Geometry: final body of the model. Coordinates: model frame, mm. A direction names the side the tool comes from. Coordinates: 2 decimals unless noted, no trailing zeros. Loops run counter-clockwise (first coordinate to the right, second up) from the corner with the lowest first, then second, coordinate; pieces in that order, holes last. Notation, with made-up numbers: (35, 47) -> (78, 47) arc R12 ccw to (78, 62) -> close; hole circle Ø2 at (25.5, 1.5). An arc over 180 degrees is marked (long way). One line per item, written item: value. Start each with the question number.
from build123d import *

# Parameters (mm, degrees)
F0_R     = 67.691
F1_DEPTH = 98.298
F2_R     = 76.523192
F3_DEPTH = 228.6


with BuildPart() as f1:
    # F0 (on Top) → F1 (new body)
    with BuildSketch(Plane.XY):
        Polygon((20.642572, -144.15397), (135.162286, -54.199993), (114.519714, 89.953977), (-20.642572, 144.15397), (-135.162286, 54.199993), (-114.519714, -89.953977), align=None)
        Circle(F0_R, mode=Mode.SUBTRACT)
    extrude(amount=F1_DEPTH)

    # F2 (on Top) → F3 (join)
    with BuildSketch(Plane.XY):
        with BuildLine():
            ThreePointArc((246.963915, -59.370235), (252.234845, -29.892856), (254, 0))
            ThreePointArc((254, 0), (251.607755, 34.778404), (244.476083, 68.901703))
            ThreePointArc((244.476083, 68.901703), (227.114105, 77.709336), (235.441325, 95.306781))
            ThreePointArc((235.441325, 95.306781), (203.739291, 151.678282), (158.82823, 198.216027))
            ThreePointArc((158.82823, 198.216027), (139.581788, 195.285642), (136.12364, 214.444293))
            ThreePointArc((136.12364, 214.444293), (77.552803, 241.870963), (13.953987, 253.616416))
            ThreePointArc((13.953987, 253.616416), (0, 240.040742), (-13.953987, 253.616416))
            ThreePointArc((-13.953987, 253.616416), (-86.873116, 238.681926), (-152.332115, 203.250896))
            ThreePointArc((-152.332115, 203.250896), (-150.086276, 199.168943), (-149.308795, 194.575289))
            ThreePointArc((-149.308795, 194.575289), (-158.313913, 181.524718), (-173.710864, 185.311996))
            ThreePointArc((-173.710864, 185.311996), (-214.880552, 135.433926), (-242.118892, 76.77527))
            ThreePointArc((-242.118892, 76.77527), (-234.821293, 71.757087), (-232.011792, 63.358051))
            ThreePointArc((-232.011792, 63.358051), (-237.268803, 52.4433), (-249.080289, 49.749468))
            ThreePointArc((-249.080289, 49.749468), (-253.570272, -14.768787), (-241.620537, -78.329536))
            ThreePointArc((-241.620537, -78.329536), (-228.899573, -80.082867), (-222.993203, -91.485142))
            ThreePointArc((-222.993203, -91.485142), (-225.333207, -99.221668), (-231.568706, -104.364431))
            ThreePointArc((-231.568706, -104.364431), (-197.704688, -159.46428), (-151.022883, -204.225583))
            ThreePointArc((-151.022883, -204.225583), (-135.388346, -198.897355), (-125.616022, -212.213904))
            ThreePointArc((-125.616022, -212.213904), (-126.148708, -216.033334), (-127.706111, -219.561265))
            ThreePointArc((-127.706111, -219.561265), (-68.115844, -244.696203), (-4.109422, -253.966755))
            ThreePointArc((-4.109422, -253.966755), (9.307669, -239.86022), (23.777564, -252.884613))
            ThreePointArc((23.777564, -252.884613), (86.873116, -238.681926), (144.336425, -209.004776))
            ThreePointArc((144.336425, -209.004776), (147.049089, -189.726443), (166.394684, -191.908336))
            ThreePointArc((166.394684, -191.908336), (209.467451, -143.664146), (238.959818, -86.105781))
            ThreePointArc((238.959818, -86.105781), (229.956513, -68.844461), (246.963915, -59.370235))
        make_face()
        Circle(F2_R, mode=Mode.SUBTRACT)
    extrude(amount=F3_DEPTH)


solid = f1.part
1. Draft query along X for faces 1 (the face through (53, 60, 228.6)), 2 (the face through (-214.395, 136.201, 112.7)), 3 (the face through (9.006, -239.875, 112.7)). Return one class per face: released by +X, released by -X, zero draft, split by the parting line, or undercut.
2. Line query: L1, parallel to X at y = 0, z = 173; L2, parallel to Y at x = 0, z = 155; L3, parallel to X at y = -19, z = 76. Output: solid intervals per line, ascending. Write a range as [from, to].
3. Section C-C on x = 116. Return the cut outline in (y, z), plus the area to 3 significant figures.
4. Set-up query: faces 4 (the face through (5, -68, 98.298)), 5 (the face through (0.302, 240.044, 112.7)). Return all of +Z, -Z, +X, -X, +Y, -Y with unobstructed straight access to the full face (end or side cutting, diameter ignored); none if empty.
5. Section B-B on y = -31. Return the cut outline in (x, z).
6. Section A-A on z = 47. Return the cut outline in (x, y).
7. Pin query (flat end, axial travel): pin 1 Ø3 at (y, z) = (-97.5, 37.5) entering from -X; pin 2 Ø10 at (y, z) = (150, 102) entering from +X; pin 3 Ø4 at (x, z) = (-132.5, 132) entering from -Y. Return the tip coordinate at first contact, or that it passes through.
8. Section D-D on y = 102. Return the cut outline in (x, z).
Checks:
1. face 1: zero draft
1. face 2: released by -X
1. face 3: undercut
2. L1: [-254, -76.52], [76.52, 254]
2. L2: [-243.92, -76.52], [76.52, 240.04]
2. L3: [-253.29, -64.97], [64.97, 253.29]
3. outline: (-225.96, 0) -> (225.96, 0) -> (225.96, 228.6) -> (-225.96, 228.6) -> close
3. area: 103,000 mm²
4. face 4: +Z
4. face 5: +Z, -Z, +Y
5. outline: (-252.1, 0) -> (-60.18, 0) -> (-60.18, 98.3) -> (-69.96, 98.3) -> (-69.96, 228.6) -> (-252.1, 228.6) -> close; (60.18, 0) -> (252.1, 0) -> (252.1, 228.6) -> (69.96, 228.6) -> (69.96, 98.3) -> (60.18, 98.3) -> close
6. outline: (-249.08, 49.75) arc R254 ccw to (-241.62, -78.33) arc R13.96 cw to (-222.99, -91.49) arc R13.96 cw to (-231.57, -104.36) arc R254 ccw to (-151.02, -204.23) arc R13.96 cw to (-125.62, -212.21) arc R13.96 cw to (-127.71, -219.56) arc R254 ccw to (-4.11, -253.97) arc R13.96 cw to (23.78, -252.88) arc R254 ccw to (144.34, -209) arc R13.96 cw to (166.39, -191.91) arc R254 ccw to (238.96, -86.11) arc R13.96 cw to (246.96, -59.37) arc R254 ccw to (254, 0) arc R254 ccw to (244.48, 68.9) arc R13.96 cw to (235.44, 95.31) arc R254 ccw to (158.83, 198.22) arc R13.96 cw to (136.12, 214.44) arc R254 ccw to (13.95, 253.62) arc R13.96 cw to (-13.95, 253.62) arc R254 ccw to (-152.33, 203.25) arc R13.96 cw to (-149.31, 194.58) arc R13.96 cw to (-173.71, 185.31) arc R254 ccw to (-242.12, 76.78) arc R13.96 cw to start; hole circle Ø135.38 at (0, 0)
7. pin 1: x = -225.19
7. pin 2: x = 208.54
7. pin 3: y = -201.61
8. outline: (-232.62, 0) -> (232.62, 0) -> (232.62, 228.6) -> (-232.62, 228.6) -> close
